from build123d import *

# Parameters (mm, degrees)
F1_DEPTH = 6.35


with BuildPart() as f1:
    # F0 (on Top) → F1 (new body)
    with BuildSketch(Plane.XY):
        Polygon((-24.1086892498, -13.7312582458), (-25.9361392682, -18.7545309792), (-20.5932268628, -18.5928845996), (-20.0483695073, -14.4970599949), align=None)
        Polygon((-16.4632104005, -18.4679336069), (-20.5932268628, -18.5928845996), (-21.2980969645, -23.8915637428), (-16.1148480755, -22.585128334), align=None)
        Polygon((-12.1082498728, -21.5752671691), (-16.1148480755, -22.585128334), (-15.6641793179, -27.9114535394), (-10.8829569025, -25.521316569), align=None)
        Polygon((-7.1871210385, -23.6737652176), (-10.8829569025, -25.521316569), (-9.2978220559, -30.6262347898), (-5.1421907603, -27.2641564062), align=None)
        Polygon((-1.9299304123, -24.665304316), (-5.1421907603, -27.2641564062), (-2.4967089684, -31.9089673401), (0.8390185068, -27.7321545918), align=None)
        Polygon((8.6051350651, -23.1959806628), (6.7809962009, -26.9034280507), (11.1322759384, -30.0081353106), (12.4059020493, -24.816727115), align=None)
        Polygon((13.3904019635, -20.8038218521), (12.4059020493, -24.816727115), (17.3228715709, -26.9134515238), (17.4507217059, -21.5696236012), align=None)
        Polygon((17.5495485484, -17.4388994534), (17.4507217059, -21.5696236012), (22.7034689817, -22.5603246559), (21.6795650107, -17.3139484608), align=None)
        Polygon((24.8946959507, -12.2486923333), (20.8880977481, -13.2585534982), (21.6795650107, -17.3139484608), (27.0224774161, -17.1523020812), align=None)
        Polygon((26.9457785766, -6.6107009659), (23.2499427125, -8.4582523173), (24.8946959507, -12.2486923333), (30.0779448398, -10.9422569245), align=None)
        Polygon((24.5246461962, -3.2624526586), (26.9457785766, -6.6107009659), (31.727000992, -4.2205639955), (27.7369065442, -0.6636005685), align=None)
        Polygon((27.2310875892, 5.3145290539), (24.6526044809, 2.0858956603), (27.7369065442, -0.6636005685), (31.8925378399, 2.6984778152), align=None)
        Polygon((23.6278343795, 7.3367098166), (27.2310875892, 5.3145290539), (30.5668150644, 9.4913418023), (25.4519732437, 11.0441572045), align=None)
        Polygon((22.4827529172, 16.2573728388), (21.498253003, 12.2444675759), (25.4519732437, 11.0441572045), (27.811821989, 15.8404011956), align=None)
        Polygon((23.7563790281, 21.4487810344), (18.4622640521, 20.710411788), (18.3634372096, 16.5796876402), (22.4827529172, 16.2573728388), align=None)
        Polygon((13.5785002392, 24.1950549), (14.3699675018, 20.1396599374), (18.4622640521, 20.710411788), (18.5901141871, 26.0542397106), align=None)
        Polygon((12.5545962682, 29.4414310951), (8.0598208465, 26.5483641356), (9.7045740847, 22.7579241196), (13.5785002392, 24.1950549), align=None)
        Polygon((2.1642731889, 27.6603013707), (4.5854055693, 24.3120530635), (8.0598208465, 26.5483641356), (5.9320393812, 31.4519738835), align=None)
        Polygon((-0.9678930743, 31.9918573294), (-3.8324734776, 27.478873656), (-0.7481714143, 24.7293774271), (2.1642731889, 27.6603013707), align=None)
        Polygon((-7.8225679254, 31.035837083), (-9.6500179437, 26.0125643496), (-6.046764734, 23.990383587), (-3.8324734776, 27.478873656), align=None)
        Polygon((-15.0163382961, 23.3299364452), (-11.0626180553, 22.1296260737), (-9.6500179437, 26.0125643496), (-14.3114681944, 28.6286155884), align=None)
        Polygon((-20.1311801167, 24.8827518473), (-19.6805113592, 19.5564266419), (-15.5611956516, 19.2341118405), (-15.0163382961, 23.3299364452), align=None)
        Polygon((-25.0095804309, 19.9733982851), (-23.4244455844, 14.8684800642), (-19.3321490342, 15.4392319148), (-19.6805113592, 19.5564266419), align=None)
        Polygon((-28.7185605604, 14.1301108179), (-26.0730787685, 9.4852998839), (-22.1991526141, 10.9224306643), (-23.4244455844, 14.8684800642), align=None)
        Polygon((-31.0846927164, 7.6261150733), (-27.5025637676, 3.6585976232), (-24.0281484903, 5.8949086953), (-26.0730787685, 9.4852998839), align=None)
        Polygon((-31.9973391892, 0.7655306637), (-27.6460594517, -2.3391765962), (-24.7336148485, 0.5917473475), (-27.5025637676, 3.6585976232), align=None)
        Polygon((-31.413825644, -6.1308491089), (-26.4968561223, -8.2275735177), (-24.2825648659, -4.7390834487), (-27.6460594517, -2.3391765962), align=None)
        Polygon((-29.3614365256, -12.7405571911), (-24.1086892498, -13.7312582458), (-22.6960891382, -9.8483199699), (-26.4968561223, -8.2275735177), align=None)
        Polygon((3.4175016151, -24.5035211982), (0.8390185068, -27.7321545918), (4.4211474556, -31.6996720419), (6.7809962009, -26.9034280507), align=None)
        Polygon((-8.8500670839, -20.754043752), (-12.1082498728, -21.5752671691), (-10.8829569025, -25.521316569), (-7.1871210385, -23.6737652176), align=None)
        Polygon((0.682293437, -22.5519066847), (-1.9299304123, -24.665304316), (0.8390185068, -27.7321545918), (3.4175016151, -24.5035211982), align=None)
        Polygon((-4.181651512, -22.1713285593), (-7.1871210385, -23.6737652176), (-5.1421907603, -27.2641564062), (-1.9299304123, -24.665304316), align=None)
        Polygon((5.5143351032, -21.8779827183), (3.4175016151, -24.5035211982), (6.7809962009, -26.9034280507), (8.6051350651, -23.1959806628), align=None)
        Polygon((10.0885325887, -20.1810685955), (8.6051350651, -23.1959806628), (12.4059020493, -24.816727115), (13.3904019635, -20.8038218521), align=None)
        Polygon((20.8880977481, -13.2585534982), (17.6299149592, -14.0797769153), (17.5495485484, -17.4388994534), (21.6795650107, -17.3139484608), align=None)
        Polygon((-27.6460594517, -2.3391765962), (-24.2825648659, -4.7390834487), (-22.4818937488, -1.9022284093), (-24.7336148485, 0.5917473475), align=None)
        Polygon((-26.4968561223, -8.2275735177), (-22.6960891382, -9.8483199699), (-21.5473566878, -6.6906979621), (-24.2825648659, -4.7390834487), align=None)
        Polygon((-22.6960891382, -9.8483199699), (-24.1086892498, -13.7312582458), (-20.0483695073, -14.4970599949), (-19.6052891763, -11.1663179144), align=None)
        Polygon((-20.0483695073, -14.4970599949), (-20.5932268628, -18.5928845996), (-16.4632104005, -18.4679336069), (-16.7465001326, -15.1198132515), align=None)
        Polygon((-13.1046633551, -18.3663229254), (-16.4632104005, -18.4679336069), (-16.1148480755, -22.585128334), (-12.1082498728, -21.5752671691), align=None)
        Polygon((14.191001503, -17.5405101349), (13.3904019635, -20.8038218521), (17.4507217059, -21.5696236012), (17.5495485484, -17.4388994534), align=None)
        Polygon((23.2499427125, -8.4582523173), (20.2444731861, -9.9606889756), (20.8880977481, -13.2585534982), (24.8946959507, -12.2486923333), align=None)
        Polygon((21.912422347, -5.3758502899), (23.2499427125, -8.4582523173), (26.9457785766, -6.6107009659), (24.5246461962, -3.2624526586), align=None)
        Polygon((24.6526044809, 2.0858956603), (22.5557709928, -0.5396428196), (24.5246461962, -3.2624526586), (27.7369065442, -0.6636005685), align=None)
        Polygon((22.1444368559, 4.3217977493), (24.6526044809, 2.0858956603), (27.2310875892, 5.3145290539), (23.6278343795, 7.3367098166), align=None)
        Polygon((21.498253003, 12.2444675759), (20.6976534634, 8.9811558587), (23.6278343795, 7.3367098166), (25.4519732437, 11.0441572045), align=None)
        Polygon((18.3634372096, 16.5796876402), (18.2830707988, 13.220565102), (21.498253003, 12.2444675759), (22.4827529172, 16.2573728388), align=None)
        Polygon((18.4622640521, 20.710411788), (14.3699675018, 20.1396599374), (15.0135920638, 16.8417954148), (18.3634372096, 16.5796876402), align=None)
        Polygon((9.7045740847, 22.7579241196), (11.0420944503, 19.6755220922), (14.3699675018, 20.1396599374), (13.5785002392, 24.1950549), align=None)
        Polygon((8.0598208465, 26.5483641356), (4.5854055693, 24.3120530635), (6.5542807727, 21.5892432244), (9.7045740847, 22.7579241196), align=None)
        Polygon((-0.7481714143, 24.7293774271), (1.7599962107, 22.4934753382), (4.5854055693, 24.3120530635), (2.1642731889, 27.6603013707), align=None)
        Polygon((-3.8324734776, 27.478873656), (-6.046764734, 23.990383587), (-3.116583818, 22.3459375448), (-0.7481714143, 24.7293774271), align=None)
        Polygon((-9.6500179437, 26.0125643496), (-11.0626180553, 22.1296260737), (-7.8474358512, 21.1535285476), (-6.046764734, 23.990383587), align=None)
        Polygon((-15.5611956516, 19.2341118405), (-12.2113505057, 18.9720040659), (-11.0626180553, 22.1296260737), (-15.0163382961, 23.3299364452), align=None)
        Polygon((-19.6805113592, 19.5564266419), (-19.3321490342, 15.4392319148), (-16.0042759826, 15.90336976), (-15.5611956516, 19.2341118405), align=None)
        Polygon((-23.4244455844, 14.8684800642), (-22.1991526141, 10.9224306643), (-19.048859302, 12.0911115594), (-19.3321490342, 15.4392319148), align=None)
        Polygon((-26.0730787685, 9.4852998839), (-24.0281484903, 5.8949086953), (-21.2027391318, 7.7134864207), (-22.1991526141, 10.9224306643), align=None)
        Polygon((-27.5025637676, 3.6585976232), (-24.7336148485, 0.5917473475), (-22.3652024449, 2.9751872298), (-24.0281484903, 5.8949086953), align=None)
    extrude(amount=F1_DEPTH)


solid = f1.part
CAD build for the part. Positions are in the model's coordinates, mm. A direction names the side the tool comes from. Coordinates: 2 decimals unless noted, no trailing zeros. Return JSON: item names as keys, results as strings.
Item 1: Probe line 1 (X direction, y = 29.5, z = 5.5); line 2 (Y direction, x = -28, z = 5.75); line 3 (Y direction, x = -27, z = 5.5). List the from-to ranges inside material, lowest first. Write a range as from..to.
Findings below:
{"line 1": "x = -8.38..-6.1, -2.55..0.83, 3.99..6.78", "line 2": "y = -13..-10.6, -7.59..-2.7, -2.09..3.34, 4.21..8.77, 12.87..14.23", "line 3": "y = -13.19..-9.02, -8.01..9.14, 11.11..14.37"}
Item 2: Which spindle directions (+Z, -Z, +X, -X, +Y, -Y) get a long thin tool onto all of the face, cutting with end or side? Do faces 3 (the flat face through (5.6, -29.3, 3.1)), 4 (the flat face through (22.199, -19.974, 3.131)), 5 (the flat face through (-24.23, 17.46, 3.13)), 6 (the flat face through (22.897, 5.85, 3.131)). Say none if no direction does.
Findings below:
{"face 3": "+Z, -Z, -Y", "face 4": "+Z, -Z, +X", "face 5": "+Z, -Z, -X", "face 6": "+Z, -Z"}
Item 3: Two-plate mould, pull along Y, no slides. Class faces 1 (the flat face through (-7.25, -28.97, 3.13)), 2 (the flat face through (23.526, -1.882, 3.131)): +Y half, -Y half, draft (parallel to the pull), parting line (faces both ways), or undercut.
Findings below:
{"face 1": "-Y half", "face 2": "undercut"}
Item 4: Drop flat-ended pins along their axis: pin 1 Ø2 at (x, z) = (-25.5, 1.5) entering from +Y; pin 2 Ø3 at (y, z) = (-8, 1) entering from +X; pin 3 Ø2 at (x, z) = (-3.5, 4) entering from +Y. Give the stop position or say it passes through.
Findings below:
{"pin 1": "stops at y = 19.97", "pin 2": "stops at x = 29.04", "pin 3": "stops at y = 29.58"}
